Design review of the part built by this model. Coordinates are the model's own, in mm. A direction names the side the tool comes from. Round coordinates to 2 decimals unless told otherwise and drop trailing zeros. Loops run counter-clockwise (first coordinate to the right, second up) from the corner with the lowest first, then second, coordinate; pieces in that order, holes last. Notation, with made-up numbers: (57.25, 32.5) - (66.25, 32.5) arc R21 ccw to (66.25, 60.5) - close; hole circle Ø5 at (83.5, 60). An arc over 180 degrees is marked (long way). Return JSON: item names as keys, results as strings. Group by question number.
from build123d import *

# Parameters (mm, degrees)
ESQUISSE1_W              = 150
ESQUISSE1_H              = 90
BOSS_EXTRU_1_DEPTH       = 2
ESQUISSE2_W              = 145
ESQUISSE2_H              = 85
ESQUISSE2_W_2            = 141
ESQUISSE2_H_2            = 81
BOSS_EXTRU_2_DEPTH       = 88
ESQUISSE3_R              = 15
ENL_V_MAT_EXTRU_1_DEPTH  = 2
ENL_V_MAT_EXTRU_2_DEPTH  = 90
ESQUISSE6_R              = 2.25
ENL_V_MAT_EXTRU_4_DEPTH  = 90
CONG_1_R                 = 2
ESQUISSE9_W              = 2
ESQUISSE9_H              = 22
BOSS_EXTRU_5_DEPTH       = 81
ESQUISSE11_W             = 3.5
ESQUISSE11_H             = 2
BOSS_EXTRU_6_DEPTH       = 12
ESQUISSE13_R             = 5.5
ENL_V_MAT_EXTRU_5_DEPTH  = 2
CONG_2_R                 = 1
ESQUISSE14_W             = 22
ESQUISSE14_H             = 2
BOSS_EXTRU_7_DEPTH       = 65
ESQUISSE16_W             = 125
ESQUISSE16_H             = 2
ENL_V_MAT_EXTRU_6_DEPTH  = 2.5
ESQUISSE18_W             = 125.5
ESQUISSE18_H             = 2
ENL_V_MAT_EXTRU_7_DEPTH  = 2.5
CONG_3_R                 = 2
ESQUISSE26_R             = 1.75
ENL_V_MAT_EXTRU_12_DEPTH = 85
ESQUISSE19_W             = 14
ESQUISSE19_H             = 10
ENL_V_MAT_EXTRU_8_DEPTH  = 2
ESQUISSE20_W             = 15.6
ESQUISSE20_H             = 14
BOSS_EXTRU_8_DEPTH       = 15
ESQUISSE23_W             = 22
ESQUISSE23_H             = 30
ENL_V_MAT_EXTRU_10_DEPTH = 44.5
ESQUISSE21_W             = 12.6
ESQUISSE21_H             = 10.4
ENL_V_MAT_EXTRU_9_DEPTH  = 15
ESQUISSE27_R             = 3.75
BOSS_EXTRU_9_DEPTH       = 4
ESQUISSE29_R             = 1.65
ENL_V_MAT_EXTRU_13_DEPTH = 4
BOSS_EXTRU_10_START      = 4
ESQUISSE30_R             = 3.75
BOSS_EXTRU_10_DEPTH      = 4
ESQUISSE31_R             = 1.65
ENL_V_MAT_EXTRU_14_DEPTH = 4
CONG_4_R                 = 2
CONG_5_R                 = 2
ESQUISSE38_W             = 13
ESQUISSE38_H             = 34
BOSS_EXTRU_13_DEPTH      = 12
ESQUISSE40_W             = 11
ESQUISSE40_H             = 32
ENL_V_MAT_EXTRU_18_DEPTH = 11.99
ESQUISSE41_W             = 9
ESQUISSE41_H             = 11.99
ENL_V_MAT_EXTRU_19_DEPTH = 1
ESQUISSE33_W             = 1
ESQUISSE33_H             = 7
ESQUISSE33_W_2           = 3
ESQUISSE33_H_2           = 1.5
BOSS_EXTRU_11_DEPTH      = 10
ENL_V_MAT_EXTRU_15_DEPTH = 1
ENL_V_MAT_EXTRU_16_DEPTH = 1
ESQUISSE36_W             = 5
ESQUISSE36_H             = 1
BOSS_EXTRU_12_DEPTH      = 10
ENL_V_MAT_EXTRU_17_DEPTH = 1


# Some blends are built 0.0001 mm under size
with BuildPart() as part:
    # Esquisse1 → Boss.-Extru.1 (new body)
    with BuildSketch(Plane.XZ):
        with Locations((75, 45)):
            Rectangle(ESQUISSE1_W, ESQUISSE1_H)
    extrude(amount=BOSS_EXTRU_1_DEPTH)

    # Esquisse2 → Boss.-Extru.2 (add)
    with BuildSketch(Plane(origin=(0, 0, 0), x_dir=(1, 0, 0), z_dir=(0, 1, 0))):
        with Locations((75, -45)):
            Rectangle(ESQUISSE2_W, ESQUISSE2_H)
        with Locations((75, -45)):
            Rectangle(ESQUISSE2_W_2, ESQUISSE2_H_2, mode=Mode.SUBTRACT)
    extrude(amount=BOSS_EXTRU_2_DEPTH)

    # Esquisse3 → Enlèv. mat.-Extru.1 (cut)
    with BuildSketch(Plane(origin=(0, 0, 0), x_dir=(1, 0, 0), z_dir=(0, 1, 0))):
        with Locations(Location((77.5, -45, 0), (0, 0, 270))):
            Circle(ESQUISSE3_R)
    extrude(amount=-ENL_V_MAT_EXTRU_1_DEPTH, mode=Mode.SUBTRACT)

    # Esquisse4 → Enlèv. mat.-Extru.2 (cut)
    with BuildSketch(Plane.XY.offset(87.5)):
        Polygon((2.5, 38), (27.5, 55), (27.5, 88), (2.5, 88), align=None)
    extrude(amount=-ENL_V_MAT_EXTRU_2_DEPTH, mode=Mode.SUBTRACT)

    # Esquisse6 → Enlèv. mat.-Extru.4 (cut)
    with BuildSketch(Plane(origin=(0, 0, 2.5), x_dir=(-1, 0, 0), z_dir=(0, 0, -1))):
        with Locations((-35, 5)):
            Circle(ESQUISSE6_R)
    extrude(amount=-ENL_V_MAT_EXTRU_4_DEPTH, mode=Mode.SUBTRACT)

    # Congé1
    cong_1_edges = [part.edges().sort_by_distance(p)[0] for p in [
        (150, -1, 0),
        (0, -1, 0),
        (0, -1, 90),
        (150, -1, 90),
    ]]
    fillet(cong_1_edges, radius=CONG_1_R)

    # Esquisse9 → Boss.-Extru.5 (add)
    with BuildSketch(Plane(origin=(0, 0, 85.5), x_dir=(-1, 0, 0), z_dir=(0, 0, -1))):
        with Locations((-27, 11)):
            Rectangle(ESQUISSE9_W, ESQUISSE9_H)
    extrude(amount=BOSS_EXTRU_5_DEPTH)

    # Esquisse11 → Boss.-Extru.6 (add)
    with BuildSketch(Plane(origin=(0, 0, 0), x_dir=(1, 0, 0), z_dir=(0, 1, 0))):
        with Locations((29.75, -57)):
            Rectangle(ESQUISSE11_W, ESQUISSE11_H)
        with Locations((29.75, -33)):
            Rectangle(ESQUISSE11_W, ESQUISSE11_H)
        Polygon((37, -32), (37, -34), (44, -34), (44, -4.5), (42, -4.5), (42, -32), align=None)
        Polygon((37, -56), (44, -56), (44, -85.5), (42, -85.5), (42, -58), (37, -58), align=None)
    extrude(amount=BOSS_EXTRU_6_DEPTH)

    # Esquisse13 → Enlèv. mat.-Extru.5 (cut)
    with BuildSketch(Plane.ZY.offset(-2.5)):
        with Locations((15.5, 29)):
            Circle(ESQUISSE13_R)
        with Locations((74.5, 29)):
            Circle(ESQUISSE13_R)
    extrude(amount=-ENL_V_MAT_EXTRU_5_DEPTH, mode=Mode.SUBTRACT)

    # Congé2
    cong_2_edges = [part.edges().sort_by_distance(p)[0] for p in [
        (4.5, 29, 10),
        (4.5, 29, 69),
    ]]
    fillet(cong_2_edges, radius=CONG_2_R)

    # Esquisse14 → Boss.-Extru.7 (add)
    with BuildSketch(Plane(origin=(0, 0, 0), x_dir=(1, 0, 0), z_dir=(0, 1, 0))):
        with Locations((134.5, -25.7)):
            Rectangle(ESQUISSE14_W, ESQUISSE14_H)
        with Locations((134.5, -68.2)):
            Rectangle(ESQUISSE14_W, ESQUISSE14_H)
    extrude(amount=BOSS_EXTRU_7_DEPTH)

    # Esquisse16 → Enlèv. mat.-Extru.6 (cut)
    with BuildSketch(Plane.XY.offset(90)):
        with Locations((77, -1)):
            Rectangle(ESQUISSE16_W, ESQUISSE16_H)
    extrude(amount=-ENL_V_MAT_EXTRU_6_DEPTH, mode=Mode.SUBTRACT)

    # Esquisse18 → Enlèv. mat.-Extru.7 (cut)
    with BuildSketch(Plane(origin=(0, 0, 0), x_dir=(-1, 0, 0), z_dir=(0, 0, -1))):
        with Locations((-77.25, -1)):
            Rectangle(ESQUISSE18_W, ESQUISSE18_H)
    extrude(amount=-ENL_V_MAT_EXTRU_7_DEPTH, mode=Mode.SUBTRACT)

    # Congé3
    cong_3_edges = [part.edges().sort_by_distance(p)[0] for p in [
        (140, -2, 1.25),
        (14.5, -2, 1.25),
        (14.5, -2, 88.75),
        (139.5, -2, 88.75),
    ]]
    fillet(cong_3_edges, radius=CONG_3_R - 0.0001)  # a hair under: the kernel refuses the full size

    # Esquisse26 → Enlèv. mat.-Extru.12 (cut)
    with BuildSketch(Plane(origin=(0, 0, 2.5), x_dir=(-1, 0, 0), z_dir=(0, 0, -1))):
        with Locations((-120, 5)):
            Circle(ESQUISSE26_R)
    extrude(amount=-ENL_V_MAT_EXTRU_12_DEPTH, mode=Mode.SUBTRACT)

    # Esquisse19 → Enlèv. mat.-Extru.8 (cut)
    with BuildSketch(Plane(origin=(28, 0, 0), x_dir=(0, 0, -1), z_dir=(1, 0, 0))):
        with Locations((-45, 5)):
            Rectangle(ESQUISSE19_W, ESQUISSE19_H)
    extrude(amount=-ENL_V_MAT_EXTRU_8_DEPTH, mode=Mode.SUBTRACT)

    # Esquisse20 → Boss.-Extru.8 (add)
    with BuildSketch(Plane(origin=(0, 0, 0), x_dir=(1, 0, 0), z_dir=(0, 1, 0))):
        with Locations((115.3, -24.4)):
            Rectangle(ESQUISSE20_W, ESQUISSE20_H)
        with Locations((115.3, -52.37)):
            Rectangle(ESQUISSE20_W, ESQUISSE20_H)
    extrude(amount=BOSS_EXTRU_8_DEPTH)

    # Esquisse23 → Enlèv. mat.-Extru.10 (cut)
    with BuildSketch(Plane(origin=(0, 0, 24.7), x_dir=(-1, 0, 0), z_dir=(0, 0, -1))):
        with Locations((-134.5, 35)):
            Rectangle(ESQUISSE23_W, ESQUISSE23_H)
    extrude(amount=-ENL_V_MAT_EXTRU_10_DEPTH, mode=Mode.SUBTRACT)

    # Esquisse21 → Enlèv. mat.-Extru.9 (cut)
    with BuildSketch(Plane(origin=(0, 15, 0), x_dir=(1, 0, 0), z_dir=(0, 1, 0))):
        with Locations((115.8, -24.4)):
            Rectangle(ESQUISSE21_W, ESQUISSE21_H)
        with Locations((115.8, -52.37)):
            Rectangle(ESQUISSE21_W, ESQUISSE21_H)
    extrude(amount=-ENL_V_MAT_EXTRU_9_DEPTH, mode=Mode.SUBTRACT)

    # Esquisse27 → Boss.-Extru.9 (add)
    with BuildSketch(Plane.XY.offset(4.5)):
        with Locations((120, 5)):
            Circle(ESQUISSE27_R)
    extrude(amount=BOSS_EXTRU_9_DEPTH)

    # Esquisse29 → Enlèv. mat.-Extru.13 (cut)
    with BuildSketch(Plane.XY.offset(8.5)):
        with Locations((120, 5)):
            Circle(ESQUISSE29_R)
    extrude(amount=-ENL_V_MAT_EXTRU_13_DEPTH, mode=Mode.SUBTRACT)

    # Esquisse30 → Boss.-Extru.10 (add)
    with BuildSketch(Plane(origin=(0, 0, 85.5), x_dir=(-1, 0, 0), z_dir=(0, 0, -1)).offset(BOSS_EXTRU_10_START)):
        with Locations(Location((-120, 5, 0), (0, 0, 180))):
            Circle(ESQUISSE30_R)
    extrude(amount=-BOSS_EXTRU_10_DEPTH)

    # Esquisse31 → Enlèv. mat.-Extru.14 (cut)
    with BuildSketch(Plane.XY.offset(85.5)):
        with Locations((120, 5)):
            Circle(ESQUISSE31_R)
    extrude(amount=-ENL_V_MAT_EXTRU_14_DEPTH, mode=Mode.SUBTRACT)

    # Congé4
    # the kernel refuses this fillet: 2 mm, written as the material it adds along each edge
    with BuildSketch(Plane(origin=(120, 5, 85.5), x_dir=(1, 0, 0), z_dir=(0, 1, 0))) as cong_4_piece_1:
        with BuildLine():
            CenterArc((3.75 + CONG_4_R, CONG_4_R), CONG_4_R, 180, 90)
            Line((3.75, CONG_4_R), (3.75, 0))
            Line((3.75, 0), (3.75 + CONG_4_R, 0))
        make_face()
    revolve(axis=Axis((120, 5, 85.5), (0, 0, -1)))

    # Congé5
    # the kernel refuses this fillet: 2 mm, written as the material it adds along each edge
    with BuildSketch(Plane(origin=(120, 5, 4.5), x_dir=(1, 0, 0), z_dir=(0, -1, 0))) as cong_5_piece_1:
        with BuildLine():
            CenterArc((3.75 + CONG_5_R, CONG_5_R), CONG_5_R, 180, 90)
            Line((3.75, CONG_5_R), (3.75, 0))
            Line((3.75, 0), (3.75 + CONG_5_R, 0))
        make_face()
    revolve(axis=Axis((120, 5, 4.5), (0, 0, 1)))

    # Esquisse38 → Boss.-Extru.13 (add)
    with BuildSketch(Plane(origin=(0, 0, 0), x_dir=(1, 0, 0), z_dir=(0, 1, 0))):
        with Locations((98, -41.5)):
            Rectangle(ESQUISSE38_W, ESQUISSE38_H)
    extrude(amount=BOSS_EXTRU_13_DEPTH)

    # Esquisse40 → Enlèv. mat.-Extru.18 (cut)
    with BuildSketch(Plane(origin=(0, 12, 0), x_dir=(1, 0, 0), z_dir=(0, 1, 0))):
        with Locations((98, -41.5)):
            Rectangle(ESQUISSE40_W, ESQUISSE40_H)
    extrude(amount=-ENL_V_MAT_EXTRU_18_DEPTH, mode=Mode.SUBTRACT)

    # Esquisse41 → Enlèv. mat.-Extru.19 (cut)
    with BuildSketch(Plane.XY.offset(25.5)):
        with Locations((98, 6.005)):
            Rectangle(ESQUISSE41_W, ESQUISSE41_H)
    extrude(amount=-ENL_V_MAT_EXTRU_19_DEPTH, mode=Mode.SUBTRACT)

    # Esquisse33 → Boss.-Extru.11 (add)
    with BuildSketch(Plane(origin=(0, 0, 0), x_dir=(1, 0, 0), z_dir=(0, 1, 0))):
        with Locations((62.5, -8)):
            Rectangle(ESQUISSE33_W, ESQUISSE33_H)
        with Locations((136, -8)):
            Rectangle(ESQUISSE33_W, ESQUISSE33_H)
        with Locations((136, -21.2)):
            Rectangle(ESQUISSE33_W, ESQUISSE33_H)
        with Locations((136, -72.7)):
            Rectangle(ESQUISSE33_W, ESQUISSE33_H)
        with Locations((136, -82)):
            Rectangle(ESQUISSE33_W, ESQUISSE33_H)
        with Locations((62.5, -82)):
            Rectangle(ESQUISSE33_W, ESQUISSE33_H)
        with Locations((106, -53.62)):
            Rectangle(ESQUISSE33_W_2, ESQUISSE33_H_2)
        with Locations((106, -29.15)):
            Rectangle(ESQUISSE33_W_2, ESQUISSE33_H_2)
    extrude(amount=BOSS_EXTRU_11_DEPTH)

    # Esquisse34 → Enlèv. mat.-Extru.15 (cut)
    with BuildSketch(Plane.ZY.offset(-62)):
        Polygon((4.5, 10), (11.5, 0), (11.5, 10), align=None)
        Polygon((85.5, 10), (78.5, 0), (78.5, 10), align=None)
    extrude(amount=-ENL_V_MAT_EXTRU_15_DEPTH, mode=Mode.SUBTRACT)

    # Esquisse35 → Enlèv. mat.-Extru.16 (cut)
    with BuildSketch(Plane.ZY.offset(-135.5)):
        Polygon((4.5, 10), (11.5, 0), (11.5, 10), align=None)
        Polygon((24.7, 10), (17.7, 0), (17.7, 10), align=None)
        Polygon((69.2, 10), (76.2, 0), (76.2, 10), align=None)
        Polygon((85.5, 10), (78.5, 0), (78.5, 10), align=None)
    extrude(amount=-ENL_V_MAT_EXTRU_16_DEPTH, mode=Mode.SUBTRACT)

    # Esquisse36 → Boss.-Extru.12 (add)
    with BuildSketch(Plane.ZY.offset(-145.5)):
        with Locations((22.2, 57)):
            Rectangle(ESQUISSE36_W, ESQUISSE36_H)
        with Locations((71.7, 57)):
            Rectangle(ESQUISSE36_W, ESQUISSE36_H)
    extrude(amount=BOSS_EXTRU_12_DEPTH)

    # Esquisse37 → Enlèv. mat.-Extru.17 (cut)
    with BuildSketch(Plane(origin=(0, 57.5, 0), x_dir=(1, 0, 0), z_dir=(0, 1, 0))):
        Polygon((145.5, -19.7), (135.5, -24.7), (135.5, -19.7), align=None)
        Polygon((145.5, -74.2), (135.5, -69.2), (135.5, -74.2), align=None)
    extrude(amount=-ENL_V_MAT_EXTRU_17_DEPTH, mode=Mode.SUBTRACT)


solid = part.part
Q1. For line 1 (Z direction, x = 139, y = 58.5); line 2 (X direction, y = 18, z = 35); line 3 (Z direction, x = 85, y = 23.5), list the stretches that pass through material, from the lowest coordinate up.
Q2. Add section C-C, the plane y = 29. State the section outline as (x, z) points, plus the area to 3 significant figures.
Q3. Insertion check: pin 1 Ø3.5 at (y, z) = (3.5, 74) entering from +X; pin 2 Ø1 at (x, y) = (29.5, 4.5) entering from +Z; pin 3 Ø1 at (y, z) = (25, 33.5) entering from -X; pin 4 Ø17.5 at (y, z) = (6.5, 56) entering from -X. Each pin has a flat end and moves straight along its axis. Give the tip position at first contact, or say it passes through.
Q4. Add section B-B, the plane x = 77.5. State the section outline as (y, z) points, plus the area to 3 significant figures.
Q5. Add section D-D, the plane z = 15.5. State the section outline as (x, y) points, plus the area to 3 significant figures.
Q6. Add section A-A, the plane x = 35. State the section outline as (y, z) points.
Q7. Tool access review of faces 1 (the cylindrical face through (121.524, 4.368, 83.528)), 2 (the flat face through (40, 6, 58)), 3 (the cylindrical face through (2.993, 34.453, 14.784)), 4 (the flat face through (134, 57, 26.7)): name each direction out of +Z, -Z, +X, -X, +Y, -Y from which nothing blocks a thin tool from reaching the whole face with its end or side.
Q8. Draft analysis for pull direction Y (two halves, no side actions). For faces 5 (the flat face through (134, 57, 69.2)), 6 (the flat face through (30, 6, 58)), 7 (the flat face through (3.831, 38.905, 45.198)), state which applies: pulls with the +Y half, pulls with the -Y half, needs draft (parallel to the pull), parting line crosses it, or undercut.
Evaluation:
{
 "1": {"line 1": "2.5 to 4.5, 24.7 to 26.7, 67.2 to 69.2, 85.5 to 87.5", "line 2": "2.5 to 4.5, 26 to 28, 145.5 to 147.5", "line 3": "2.5 to 4.5, 85.5 to 87.5"},
 "2": {"outline": "(2.5, 2.5) - (147.5, 2.5) - (147.5, 87.5) - (2.5, 87.5) - (2.5, 80) - (3.5, 80) arc R1 ccw to (4.5, 81) - (4.5, 85.5) - (145.5, 85.5) - (145.5, 4.5) - (4.5, 4.5) - (4.5, 9) arc R1 ccw to (3.5, 10) - (2.5, 10) - close; (2.5, 21) - (3.5, 21) arc R1 ccw to (4.5, 22) - (4.5, 68) arc R1 ccw to (3.5, 69) - (2.5, 69) - close", "area": "859 mm²"},
 "3": {"pin 1": "x = 147.5", "pin 2": "z = 87.5", "pin 3": "x = 2.5", "pin 4": "x = 0"},
 "4": {"outline": "(-2, 2.5) - (88, 2.5) - (88, 4.5) - (0, 4.5) - (0, 30) - (-2, 30) - close; (-2, 60) - (0, 60) - (0, 85.5) - (88, 85.5) - (88, 87.5) - (-2, 87.5) - close", "area": "462 mm²"},
 "5": {"outline": "(0, -2) - (150, -2) - (150, 0) - (147.5, 0) - (147.5, 88) - (145.5, 88) - (145.5, 0) - (44, 0) - (44, 12) - (42, 12) - (42, 0) - (28, 0) - (28, 22) - (26, 22) - (26, 0) - (4.5, 0) - (4.5, 22.5) arc R1 ccw to (3.5, 23.5) - (2.5, 23.5) - (2.5, 0) - (0, 0) - close; (2.5, 34.5) - (3.5, 34.5) arc R1 ccw to (4.5, 35.5) - (4.5, 39.36) - (2.5, 38) - close", "area": "599 mm²"},
 "6": {"outline": "(-2, 2.5) - (2.75, 2.5) - (2.75, 4.5) - (0, 4.5) - (0, 85.5) - (2.75, 85.5) - (2.75, 87.5) - (-2, 87.5) - close; (7.25, 2.5) - (88, 2.5) - (88, 4.5) - (7.25, 4.5) - close; (7.25, 85.5) - (88, 85.5) - (88, 87.5) - (7.25, 87.5) - close"},
 "7": {"face 1": "+Z", "face 2": "+Y", "face 3": "-X", "face 4": "-X, +Y"},
 "8": {"face 5": "undercut", "face 6": "needs draft", "face 7": "pulls with the +Y half"}
}
